Here's how the part is built. I have some questions about the finished solid (model axes, mm). Coordinates: 2 decimals unless noted, no trailing zeros. Loops run counter-clockwise (first coordinate to the right, second up) from the corner with the lowest first, then second, coordinate; pieces in that order, holes last. Notation, with made-up numbers: (-29, 4) -> (-24, 4) arc R13 ccw to (-24, 14) -> close; hole circle Ø10 at (71, -11.5). An arc over 180 degrees is marked (long way). Answer as a JSON object with one key per item and string values. Group by question number.
Q1. I want a section at B-B on z = 0.25. Write out the boundary of the cut face in (x, y), then the cut area to 3 significant figures.
Q2. I need wall thicknesses on line 1 (Z direction, x = 4.4, y = 2.5); line 2 (X direction, y = 1.5, z = 0.35); line 3 (X direction, y = 1, z = 0.1). Which ranges of each line are inside material? Lowest first, please.
Q3. I want a section at A-A on y = 6.5. Write out the boundary of the cut face in (x, z).
```python
from build123d import *

# Parameters (mm, degrees)
EXTRUDE_1_DEPTH = 8


with BuildPart() as part:
    # 草图1 → 凸台-拉伸1 (new body)
    with BuildSketch(Plane(origin=(0, 0, 0), x_dir=(1, 0, 0), z_dir=(0, 1, 0))):
        with BuildLine():
            Line((4.181064308, -0.346153929), (4.266632429, -0.111057449))
            ThreePointArc((4.266632429, -0.111057449), (4.413078903, 0.079795311), (4.642509478, 0.152134494))
            Line((4.642509478, 0.152134494), (4.697815899, 0.152134494))
            Line((4.697815899, 0.152134494), (4.697815899, 0.43758725))
            Line((4.697815899, 0.43758725), (2.568518685, 0.43758725))
            Line((2.568518685, 0.43758725), (2.568518685, 0.152134494))
            Line((2.568518685, 0.152134494), (2.623825106, 0.152134494))
            ThreePointArc((2.623825106, 0.152134494), (2.853255681, 0.079795311), (2.999702154, -0.111057449))
            Line((2.999702154, -0.111057449), (3.085270275, -0.346153929))
            ThreePointArc((3.085270275, -0.346153929), (3.158493512, -0.441580309), (3.273208799, -0.477749901))
            Line((3.273208799, -0.477749901), (3.993125784, -0.477749901))
            ThreePointArc((3.993125784, -0.477749901), (4.107841071, -0.441580309), (4.181064308, -0.346153929))
        make_face()
    extrude(amount=EXTRUDE_1_DEPTH)


solid = part.part
```
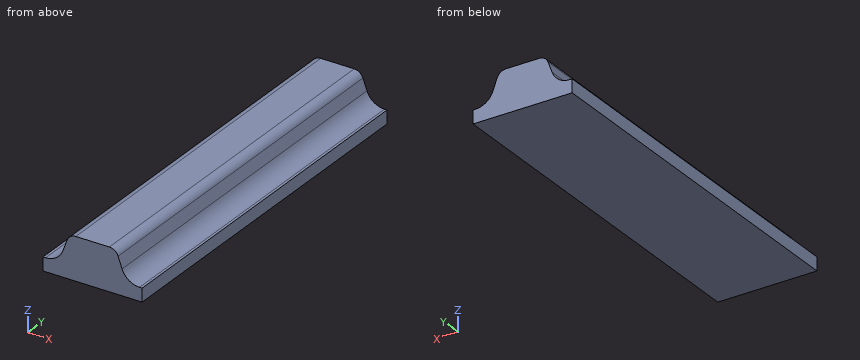
Result set:
{
 "1": {"outline": "(3.05, 0) -> (4.22, 0) -> (4.22, 8) -> (3.05, 8) -> close", "area": "9.33 mm²"},
 "2": {"line 1": "z = -0.44 to -0.07", "line 2": "x = 3.09 to 4.18", "line 3": "x = 3 to 4.27"},
 "3": {"outline": "(2.57, -0.44) -> (4.7, -0.44) -> (4.7, -0.15) -> (4.64, -0.15) arc R0.4 cw to (4.27, 0.11) -> (4.18, 0.35) arc R0.2 ccw to (3.99, 0.48) -> (3.27, 0.48) arc R0.2 ccw to (3.09, 0.35) -> (3, 0.11) arc R0.4 cw to (2.62, -0.15) -> (2.57, -0.15) -> close"}
}
